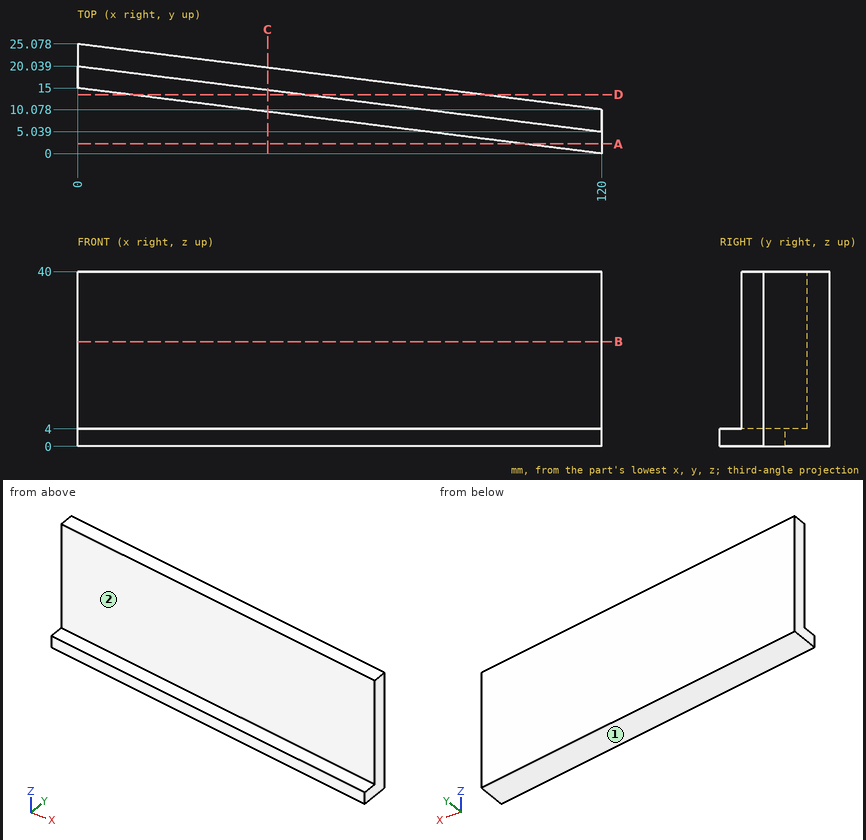
Verification items for this drawing (mm, ordinates from the low corner). A direction names the side the tool comes from. Coordinates: 2 decimals unless noted, no trailing zeros. Write each loop counter-clockwise with the first axis right and the second up, starting at its lowest first coordinate (ties: lowest second). Pieces come first, ordered by that corner, then holes. Notation, with made-up numbers: (-36.75, -33) -> (1.25, -33) arc R31 cw to (1.25, 2) -> close; hole circle Ø11 at (43.5, 44.5). An arc over 180 degrees is marked (long way). Use CSV: the item, a comma, the result in double quotes. Start each with the question number.
Item 1: Depth check by flat-ended pin: pin 1 Ø4 at (x, y) = (62.5, 21) entering from -Z; pin 2 Ø12 at (x, y) = (101.5, 7) entering from -Z; pin 3 Ø12 at (x, y) = (59.5, 5) entering from +Z; pin 4 Ø2 at (x, z) = (81, 5) entering from +Y. Enter the tip coordinate at first touch or a pass-through.
Item 2: Cross-section at C-C, the plane x = 43.5. Record the cut outline in (y, z).
Item 3: Set-up check for the marked faces 1 and 2: record each of +Z, -Z, +X, -X, +Y, -Y from which the full face is reachable in a straight line by a thin tool's end or side.
Item 4: Cross-section at A-A, the plane y = 2.25. Record the cut outline in (x, z), plus the area to 3 significant figures.
Item 5: Cross-section at B-B, the plane z = 24. Record the cut outline in (x, y), plus the area to 3 significant figures.
Item 6: Thickness scan on line 1 (Z direction, x = 114, y = 3.75); line 2 (Y direction, x = 79, z = 10); line 3 (Y direction, x = 26, z = 38). Record the ranges inside material, lowest first.
Item 7: Cross-section at D-D, the plane y = 13.5. Record the cut outline in (x, z).
Answers:
1,pin 1,"through"
1,pin 2,"z = 0"
1,pin 3,"z = 4"
1,pin 4,"y = 15.08"
2,outline,"(9.56, 0) -> (19.64, 0) -> (19.64, 40) -> (14.6, 40) -> (14.6, 4) -> (9.56, 4) -> close"
3,face 1,"-Z, +X, -X, +Y, -Y"
3,face 2,"+Z, -X, -Y"
4,outline,"(102, 0) -> (120, 0) -> (120, 4) -> (102, 4) -> close"
4,area,"72.0 mm^2"
5,outline,"(0, 20.04) -> (120, 5.04) -> (120, 10.08) -> (0, 25.08) -> close"
5,area,"605 mm^2"
6,line 1,"0 to 4"
6,line 2,"10.16 to 15.2"
6,line 3,"16.79 to 21.83"
7,outline,"(12, 0) -> (92.62, 0) -> (92.62, 40) -> (52.31, 40) -> (52.31, 4) -> (12, 4) -> close"
